Part model, mm, in its own coordinate system. Face numbers are marked on the shaded views. A direction names the side the tool comes from. Give positions to 0.01 mm unless a question says otherwise; leave off trailing zeros. Order: outer loops, then holes, each group sorted by start corner. A loop starts at its lowest first (then second) coordinate and runs counter-clockwise, first axis right, second up. Notation, with made-up numbers: M 43,44.25 L 47,44.25 A26 cw 47,69.25 Z; hole C 3.5,48 d3. An arc over 180 degrees is marked long. One line per question, with ' | ' between items.
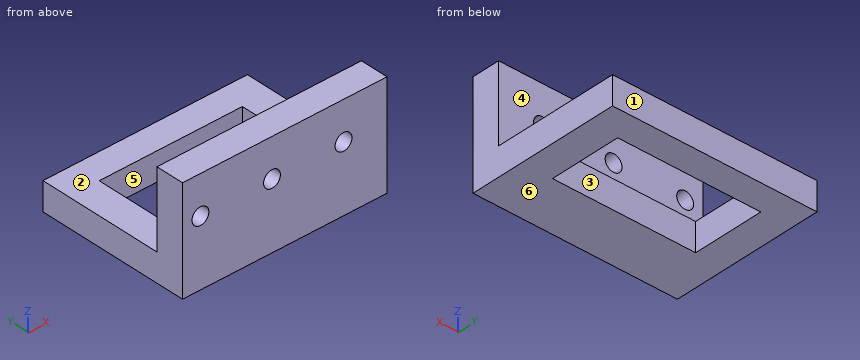
```python
from build123d import *

# Parameters (mm, degrees)
SKETCH1_W           = 40
SKETCH1_H           = 30
BOSS_EXTRUDE1_DEPTH = 5.5
SKETCH4_W           = 28
SKETCH4_H           = 14
CUT_EXTRUDE1_DEPTH  = 5.5
SKETCH5_W           = 40
SKETCH5_H           = 5.5
BOSS_EXTRUDE2_DEPTH = 15
SKETCH6_R           = 1.65
CUT_EXTRUDE3_DEPTH  = 15


with BuildPart() as part:
    # Sketch1 → Boss-Extrude1 (new body)
    with BuildSketch(Plane.XY):
        with Locations((-0.222222222, -4.277777778)):
            Rectangle(SKETCH1_W, SKETCH1_H)
    extrude(amount=BOSS_EXTRUDE1_DEPTH)

    # Sketch4 → Cut-Extrude1 (cut)
    with BuildSketch(Plane.XY.offset(5.5)):
        with Locations((-0.222222222, -1.777777778)):
            Rectangle(SKETCH4_W, SKETCH4_H)
    extrude(amount=-CUT_EXTRUDE1_DEPTH, mode=Mode.SUBTRACT)

    # Sketch5 → Boss-Extrude2 (add)
    with BuildSketch(Plane.XY.offset(5.5)):
        with Locations((-0.222222222, -16.527777778)):
            Rectangle(SKETCH5_W, SKETCH5_H)
    extrude(amount=BOSS_EXTRUDE2_DEPTH)

    # Sketch6 → Cut-Extrude3 (cut)
    with BuildSketch(Plane.XZ.offset(19.277777778)):
        with Locations(Location((-16.722222222, 13, 0), (0, 0, 270))):
            Circle(SKETCH6_R)
        with Locations(Location((-2.722222222, 13, 0), (0, 0, 270))):
            Circle(SKETCH6_R)
        with Locations(Location((11.277777778, 13, 0), (0, 0, 270))):
            Circle(SKETCH6_R)
    extrude(amount=-CUT_EXTRUDE3_DEPTH, mode=Mode.SUBTRACT)


solid = part.part
```
1. Slice it at B-B on y = -3.75. Give the cut face in (x, z).
Worked out:
outline: M -20.22,0 L -14.22,0 L -14.22,5.5 L -20.22,5.5 Z; M 13.78,0 L 19.78,0 L 19.78,5.5 L 13.78,5.5 Z
2. Mould opens along Y. For the marked faces 4, 5 and 6 say: released by +Y, released by -Y, zero draft, split by the parting line, or undercut.
Worked out:
face 4: released by +Y | face 5: undercut | face 6: zero draft
3. Slice it at D-D on z = 13. Give the cut face in (x, y), then the cut area to 3 significant figures.
Worked out:
outline: M -20.22,-19.28 L -18.37,-19.28 L -18.37,-13.78 L -20.22,-13.78 Z; M -15.07,-19.28 L -4.37,-19.28 L -4.37,-13.78 L -15.07,-13.78 Z; M -1.07,-19.28 L 9.63,-19.28 L 9.63,-13.78 L -1.07,-13.78 Z; M 12.93,-19.28 L 19.78,-19.28 L 19.78,-13.78 L 12.93,-13.78 Z | area: 166 mm2
4. Probe L1, parallel to Y at x = -8, z = 1; L2, parallel to X at y = -17, z = 13; L3, parallel to X at y = 1.75, z = 2.25. List the from-to ranges inside material, lowest first. Write a range as from..to.
Worked out:
L1: y = -19.28..-8.78, 5.22..10.72 | L2: x = -20.22..-18.37, -15.07..-4.37, -1.07..9.63, 12.93..19.78 | L3: x = -20.22..-14.22, 13.78..19.78
5. Tool access for the marked faces 1, 2 and 3: list every direction of +Z, -Z, +X, -X, +Y, -Y with a clear straight run to the whole face (end or side of a thin tool).
Worked out:
face 1: +Z, -Z, +X, -X, +Y | face 2: +Z, +X, -X, +Y | face 3: +Z, -Z
6. Drop flat-ended pins along their axis: pin 1 (10 mm diameter, centred on y = -1.5, z = 14, fed in from -X); pin 2 (4.5 mm diameter, centred on x = -3, z = 16, fed in from +Y). Give the stop position or say it passes through.
Worked out:
pin 1: passes through | pin 2: stops at y = -13.78
7. Slice it at A-A on z = 2.75. Give the cut face in (x, y).
Worked out:
outline: M -20.22,-19.28 L 19.78,-19.28 L 19.78,10.72 L -20.22,10.72 Z; hole M -14.22,-8.78 L 13.78,-8.78 L 13.78,5.22 L -14.22,5.22 Z
8. Slice it at C-C on x = -6.5. Give the cut face in (y, z), then the cut area to 4 significant figures.
Worked out:
outline: M -19.28,0 L -8.78,0 L -8.78,5.5 L -13.78,5.5 L -13.78,20.5 L -19.28,20.5 Z; M 5.22,0 L 10.72,0 L 10.72,5.5 L 5.22,5.5 Z | area: 170.5 mm2
